Read the model definition and answer for the solid it produces. Units are mm, in the model's axes. A direction names the side the tool comes from. Coordinates: 2 decimals unless noted, no trailing zeros. Order: outer loops, then holes, each group sorted by start corner. A loop starts at its lowest first (then second) coordinate and runs counter-clockwise, first axis right, second up.
from build123d import *

# Parameters (mm, degrees)
F0_W     = 600
F0_H     = 939.8
F1_DEPTH = 177.8
F2_W     = 561.9
F2_H     = 431.8
F2_H_2   = 450.85
F3_DEPTH = 355.601
F4_W     = 600
F4_H     = 965.2
F5_DEPTH = 3.175
F7_DEPTH = 19.05


with BuildPart() as f1:
    # F0 (on Front) → F1 (new body, symmetric)
    with BuildSketch(Plane.XZ):
        Rectangle(F0_W, F0_H)
    extrude(amount=F1_DEPTH, both=True)

    # F2 (on face) → F3 (cut, through all)
    with BuildSketch(Plane.XZ.offset(177.8)):
        with Locations((0, 234.95)):
            Rectangle(F2_W, F2_H)
        with Locations((0, -225.425)):
            Rectangle(F2_W, F2_H_2)
    extrude(amount=-F3_DEPTH, mode=Mode.SUBTRACT)

    # F4 (on face) → F5 (join, symmetric)
    with BuildSketch(Plane(origin=(0, 177.8, 0), x_dir=(-1, 0, 0), z_dir=(0, 1, 0))):
        with Locations((0, 12.7)):
            Rectangle(F4_W, F4_H)
    extrude(amount=F5_DEPTH, both=True)

    # F6 (on face) → F7 (join)
    with BuildSketch(Plane.XY.offset(469.9)):
        Polygon((-350.8, 174.625), (-350.8, -231.775), (360.4, -231.775), (360.4, 174.625), (300, 174.625), (300, -177.8), (-300, -177.8), (-300, 174.625), align=None)
    extrude(amount=-F7_DEPTH)


solid = f1.part
Q1. The part is cut by section A-A, the plane y = 69. Determine the outline of the cut face in (x, z), then the cut area to 3 significant figures.
Q2. Which of the six approach directions +Z, -Z, +X, -X, +Y, -Y give full straight-line access (tool end or side, diameter ignored) to faces 4 (the flat face through (-290, -177.8, -7)), 5 (the flat face through (4, 174.625, 483)), 6 (the flat face through (4, 174.625, -222))?
Q3. Straight lines are drawn through the part: L1, parallel to Z at x = 133.5, y = -125; L2, parallel to X at y = -34, z = 238; L3, parallel to Z at x = -289, y = -104. For each, find the intervals that lie inside material, in ascending order.
Q4. The part is cut by section B-B, the plane z = 42.5. Determine the outline of the cut face in (x, y) (3 decimals), then the cut area to 3 significant figures.
Q5. Determine the mould class of faces 1 (the flat face through (-4, -4, 19.05)), 2 (the flat face through (0, -231.775, 461)), 3 (the flat face through (-350.8, -26, 461)) for opening direction X: +X half, -X half, draft (parallel to the pull), parting line (faces both ways), or undercut.
Q6. Each of these flat-tipped pins is pushed along its axis until it touches: P1, Ø12, axis at y = 85, z = 213, coming from the +X side; P2, Ø21, axis at x = -324.5, z = 457.5, coming from the +Y side (3 decimals); P3, Ø1.5, axis at y = 111, z = 135, coming from the -X side. Where does it stop, or does it pass through?
Q7. The part is cut by section C-C, the plane x = -141.5. Determine the outline of the cut face in (y, z) (3 decimals).
Computed values:
1. outline: (-350.8, 450.85) - (-300, 450.85) - (-300, -469.9) - (300, -469.9) - (300, 450.85) - (360.4, 450.85) - (360.4, 469.9) - (-350.8, 469.9) - close; hole (-280.95, -450.85) - (280.95, -450.85) - (280.95, 0) - (-280.95, 0) - close; hole (-280.95, 19.05) - (280.95, 19.05) - (280.95, 450.85) - (-280.95, 450.85) - close
1. area: 70,000 mm2
2. face 4: -Z, +X, -X, -Y
2. face 5: +Z, +X, -X, -Y
2. face 6: -Y
3. L1: z = -469.9 to -450.85, 0 to 19.05, 450.85 to 469.9
3. L2: x = -300 to -280.95, 280.95 to 300
3. L3: z = -469.9 to 469.9
4. outline: (-300, -177.8) - (-280.95, -177.8) - (-280.95, 174.625) - (280.95, 174.625) - (280.95, -177.8) - (300, -177.8) - (300, 180.975) - (-300, 180.975) - close
4. area: 17,200 mm2
5. face 1: undercut
5. face 2: draft
5. face 3: -X half
6. P1: stops at x = 300
6. P2: stops at y = 174.625
6. P3: stops at x = -300
7. outline: (-231.775, 450.85) - (174.625, 450.85) - (174.625, 19.05) - (-177.8, 19.05) - (-177.8, 0) - (174.625, 0) - (174.625, -450.85) - (-177.8, -450.85) - (-177.8, -469.9) - (180.975, -469.9) - (180.975, 495.3) - (174.625, 495.3) - (174.625, 469.9) - (-231.775, 469.9) - close
